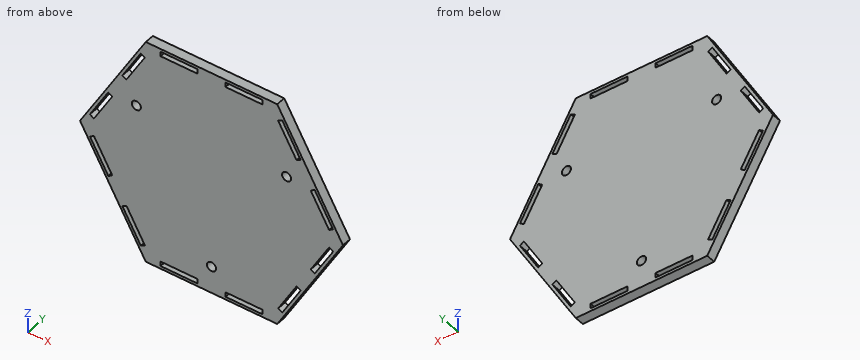
from build123d import *

# Parameters (mm, degrees)
BOSS_EXTRUDE1_DEPTH = 6.35
SKETCH2_R           = 3.0734
SKETCH2_W           = 24.892
SKETCH2_H           = 3.175
CUT_EXTRUDE1_DEPTH  = 7.35


with BuildPart() as part:
    # Sketch1 → Boss-Extrude1 (new body)
    with BuildSketch(Plane(origin=(0, 0, 0), x_dir=(1, 0, 0), z_dir=(0, 1, 0))):
        Polygon((-88.9, 0), (-44.45, -76.989658396), (44.45, -76.989658396), (88.9, 0), (44.45, 76.989658396), (-44.45, 76.989658396), align=None)
    extrude(amount=BOSS_EXTRUDE1_DEPTH)

    # Sketch2 → Cut-Extrude1 (cut, through all)
    with BuildSketch(Plane(origin=(0, 6.35, 0), x_dir=(1, 0, 0), z_dir=(0, 1, 0))):
        with Locations((-50.8, -29.329393675)):
            Circle(SKETCH2_R)
        with Locations((0, 58.65878735)):
            Circle(SKETCH2_R)
        with Locations((50.8, -29.329393675)):
            Circle(SKETCH2_R)
        Polygon((-79.484090949, -6.148832876), (-82.233721606, -7.736332876), (-69.787721606, -29.293437227), (-67.038090949, -27.705937227), align=None)
        Polygon((-45.067090949, -65.76082552), (-47.816721606, -67.34832552), (-60.262721606, -45.791221169), (-57.513090949, -44.203721169), align=None)
        Polygon((-45.067090949, 65.76082552), (-47.816721606, 67.34832552), (-60.262721606, 45.791221169), (-57.513090949, 44.203721169), align=None)
        Polygon((-69.787721606, 29.293437227), (-67.038090949, 27.705937227), (-79.484090949, 6.148832876), (-82.233721606, 7.736332876), align=None)
        with Locations((21.971, 73.497158396)):
            Rectangle(SKETCH2_W, SKETCH2_H)
        with Locations((-21.971, 73.497158396)):
            Rectangle(SKETCH2_W, SKETCH2_H)
        Polygon((79.484090949, 6.148832876), (82.233721606, 7.736332876), (69.787721606, 29.293437227), (67.038090949, 27.705937227), align=None)
        Polygon((60.262721606, 45.791221169), (57.513090949, 44.203721169), (45.067090949, 65.76082552), (47.816721606, 67.34832552), align=None)
        Polygon((45.067090949, -65.76082552), (47.816721606, -67.34832552), (60.262721606, -45.791221169), (57.513090949, -44.203721169), align=None)
        Polygon((69.787721606, -29.293437227), (67.038090949, -27.705937227), (79.484090949, -6.148832876), (82.233721606, -7.736332876), align=None)
        with Locations((-21.971, -73.497158396)):
            Rectangle(SKETCH2_W, SKETCH2_H)
        with Locations((21.971, -73.497158396)):
            Rectangle(SKETCH2_W, SKETCH2_H)
    extrude(amount=-CUT_EXTRUDE1_DEPTH, mode=Mode.SUBTRACT)


solid = part.part
Can you work these out from the model? Positions are in its coordinate system, mm. Give positions to 0.01 mm unless a question says otherwise; leave off trailing zeros. Loops run counter-clockwise (first coordinate to the right, second up) from the corner with the lowest first, then second, coordinate; pieces in that order, holes last. Notation, with made-up numbers: (34, 40) - (40, 40) arc R7 ccw to (40, 53) - close; hole circle Ø9 at (58.5, 39). An arc over 180 degrees is marked (long way). Return JSON: item names as keys, results as strings.
1. I want a section at C-C on z = -14. Please give me the cut outline in (x, y), and give its area (3 significant figures).
Output values:
{"outline": "(-80.82, 0) - (-78.62, 0) - (-78.62, 6.35) - (-80.82, 6.35) - close; (-74.95, 0) - (74.95, 0) - (74.95, 6.35) - (-74.95, 6.35) - close; (78.62, 0) - (80.82, 0) - (80.82, 6.35) - (78.62, 6.35) - close", "area": "980 mm²"}
2. If I drill on line 1 (Z direction, x = -25, y = 0.75); line 2 (Z direction, x = 50.8, y = 1.5); line 3 (X direction, y = 2, z = 60), over which ranges is the centre line in solid material (lowest first)?
Output values:
{"line 1": "z = -76.99 to -75.08, -71.91 to 71.91, 75.08 to 76.99", "line 2": "z = -65.99 to -62.18, -55.83 to 26.26, 32.4 to 55.83, 62.18 to 65.99", "line 3": "x = -54.26 to -52.06, -48.39 to 48.39, 52.06 to 54.26"}
3. I want a section at B-B on x = -32. Please give me the cut outline in (y, z), and give its area (3 significant figures).
Output values:
{"outline": "(0, -76.99) - (6.35, -76.99) - (6.35, -75.08) - (0, -75.08) - close; (0, -71.91) - (6.35, -71.91) - (6.35, 71.91) - (0, 71.91) - close; (0, 75.08) - (6.35, 75.08) - (6.35, 76.99) - (0, 76.99) - close", "area": "937 mm²"}
4. I'm going to push flat-ended pins straight in: pin 1 Ø1.6 at (y, z) = (3, -73) entering from -X; pin 2 Ø1.5 at (y, z) = (4.5, 57) entering from +X; pin 3 Ø10 at (x, z) = (-50.8, 29.33) entering from -Y; pin 4 Ø3.5 at (y, z) = (2, -73.5) entering from +X. Where does each tip first touch, or does it pass through?
Output values:
{"pin 1": "stops at x = -47.22", "pin 2": "stops at x = 56.42", "pin 3": "stops at y = 0", "pin 4": "stops at x = 47.48"}
5. I want a section at A-A on x = 0. Please give me the cut outline in (y, z), and give its area (3 significant figures).
Output values:
{"outline": "(0, -76.99) - (6.35, -76.99) - (6.35, -61.73) - (0, -61.73) - close; (0, -55.59) - (6.35, -55.59) - (6.35, 76.99) - (0, 76.99) - close", "area": "939 mm²"}
6. I want a section at D-D on x = -50.8. Please give me the cut outline in (y, z), and give its area (3 significant figures).
Output values:
{"outline": "(0, -65.99) - (6.35, -65.99) - (6.35, -62.18) - (0, -62.18) - close; (0, -55.83) - (6.35, -55.83) - (6.35, 26.26) - (0, 26.26) - close; (0, 32.4) - (6.35, 32.4) - (6.35, 55.83) - (0, 55.83) - close; (0, 62.18) - (6.35, 62.18) - (6.35, 65.99) - (0, 65.99) - close", "area": "718 mm²"}
